from build123d import *

# Parameters (mm, degrees)
SKETCH1_R           = 35
BOSS_EXTRUDE1_DEPTH = 10
CUT_EXTRUDE1_DEPTH  = 10
CIRPATTERN1_COUNT   = 18
SKETCH3_R           = 5
CUT_EXTRUDE2_DEPTH  = 10


with BuildPart() as part:
    # Sketch1 → Boss-Extrude1 (new body)
    with BuildSketch(Plane.XY):
        Circle(SKETCH1_R)
    extrude(amount=BOSS_EXTRUDE1_DEPTH)

    # Sketch2 → Cut-Extrude1 (cut)
    with BuildSketch(Plane.XY):
        with BuildLine():
            Line((0, 27.161016151), (-1.7, 27.161016151))
            ThreePointArc((-1.7, 27.161016151), (-2.629181754, 31.219024201), (-5, 34.641016151))
            ThreePointArc((-5, 34.641016151), (-2.962634917, 36.808842577), (0, 37.07925382))
            ThreePointArc((0, 37.07925382), (2.962634917, 36.808842577), (5, 34.641016151))
            ThreePointArc((5, 34.641016151), (2.629181754, 31.219024201), (1.7, 27.161016151))
            Line((1.7, 27.161016151), (0, 27.161016151))
        make_face()
    cut_extrude1 = extrude(amount=CUT_EXTRUDE1_DEPTH, mode=Mode.SUBTRACT)

    # CirPattern1: Cut-Extrude1 ×18 about axis
    cirpattern1_axis = Axis((0, 0, 0), (0, 0, 1))
    for i in range(1, CIRPATTERN1_COUNT):
        add(cut_extrude1.rotate(cirpattern1_axis, i * 360 / CIRPATTERN1_COUNT), mode=Mode.SUBTRACT)

    # Sketch3 → Cut-Extrude2 (cut)
    with BuildSketch(Plane.XY):
        Circle(SKETCH3_R)
    extrude(amount=CUT_EXTRUDE2_DEPTH, mode=Mode.SUBTRACT)


solid = part.part
Build history of the part. All positions in model axes, mm. A direction names the side the tool comes from. Round coordinates to 2 decimals unless told otherwise and drop trailing zeros. Write each loop counter-clockwise with the first axis right and the second up, starting at its lowest first coordinate (ties: lowest second). Pieces come first, ordered by that corner, then holes. Notation, with made-up numbers: M -23.75,-36.5 L 12.25,-36.5 A16 ccw 12.25,-28.5 Z; hole C 31,78 d6. An arc over 180 degrees is marked long. Answer as a JSON object with one key per item and string values. Group by question number.
(1) Cut at B-B (y = 0). Give the cut face in (x, z), and give its area (3 significant figures).
(2) Which spindle directions (+Z, -Z, +X, -X, +Y, -Y) get a long thin tool onto all of the face, cutting with end or side? Do faces 1 (the cylindrical face through (30.337, -8.043, 4.93)), 2 (the cylindrical face through (32.894, 11.956, 4.93)), 3 (the cylindrical face through (13.108, -28.395, 4.93)), 4 (the cylindrical face through (28.293, -13.326, 4.93)), 5 (the cylindrical face through (-26.82, -22.49, 4.93)). Say none if no direction does.
(3) Drill centre lines: L1, parallel to Y at x = 0, z = 7; L2, parallel to Y at x = -29, z = 5.25; L3, parallel to X at y = -27, z = 8. Where is each one in solid material? Low to high.
(4) Cut at C-C (x = 14.5). Give the cut face in (y, z), and give its area (3 significant figures).
(5) Mould opens along Y. For faces 6 (the cylindrical face through (-6.093, -34.466, 4.93)), 7 (the flat face through (0, -7, 0)), 8 (the cylindrical face through (-1.08, -4.88, 4.93)), 9 (the cylindrical face through (31.258, 2.818, 4.93)) say: pulls with the +Y half, pulls with the -Y half, needs draft (parallel to the pull), parting line crosses it, or undercut.
(6) Flat gauge pins, fed straight in: pin 1 (3 mm diameter, centred on x = 12, y = -17, fed in from -Z); pin 2 (1 mm diameter, centred on x = 0.5, z = 4.5, fed in from +Y); pin 3 (1 mm diameter, centred on x = -25.5, z = 4, fed in from +Y); pin 4 (3 mm diameter, centred on y = -10.5, z = 5.5, fed in from -X). Where does each tip first touch, or does it go through?
(7) Cut at A-A (x = 0). Give the cut face in (y, z).
Responses:
{
 "1": {"outline": "M -35,0 L -5,0 L -5,10 L -35,10 Z; M 5,0 L 35,0 L 35,10 L 5,10 Z", "area": "600 mm2"},
 "2": {"face 1": "+Z, -Z, +X", "face 2": "+Z, -Z, +X, +Y", "face 3": "+Z, -Z, -Y", "face 4": "+Z, -Z", "face 5": "+Z, -Z, -X, -Y"},
 "3": {"L1": "y = -27.16 to -5, 5 to 27.16", "L2": "y = -13.38 to -7.27, -3.14 to 3.14, 7.27 to 13.38", "L3": "x = -18.36 to -11.99, -7.94 to 7.94, 11.99 to 18.36"},
 "4": {"outline": "M -29.63,0 L 29.63,0 L 29.63,10 L -29.63,10 Z", "area": "593 mm2"},
 "5": {"face 6": "pulls with the -Y half", "face 7": "needs draft", "face 8": "undercut", "face 9": "undercut"},
 "6": {"pin 1": "stops at z = 0", "pin 2": "stops at y = 27.16", "pin 3": "stops at y = 23.31", "pin 4": "stops at x = -33.25"},
 "7": {"outline": "M -27.16,0 L -5,0 L -5,10 L -27.16,10 Z; M 5,0 L 27.16,0 L 27.16,10 L 5,10 Z"}
}
